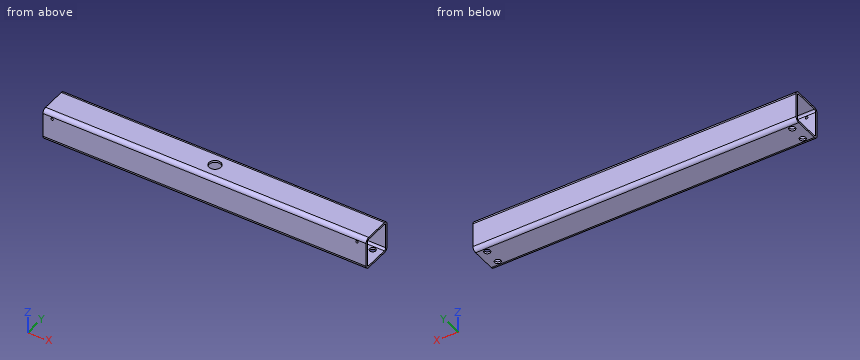
```python
from build123d import *

# Parameters (mm, degrees)
BASE_EXTRUDE_DEPTH = 511.175
SKETCH3_R          = 19.05
CUT_EXTRUDE1_DEPTH = 25.4
SKETCH4_R          = 9.525
CUT_EXTRUDE2_DEPTH = 25.4
SKETCH5_R          = 3.9751
CUT_EXTRUDE3_DEPTH = 25.4


with BuildPart() as part:
    # Sketch1 → Base-Extrude (new, symmetric)
    with BuildSketch(Plane(origin=(0, 0, 0), x_dir=(0, 0, -1), z_dir=(1, 0, 0))):
        with BuildLine():
            Line((-127, 139.7), (-50.8, 139.7))
            ThreePointArc((-50.8, 139.7), (-41.819743879, 135.980256121), (-38.1, 127))
            Line((-38.1, 127), (-38.1, 50.8))
            ThreePointArc((-38.1, 50.8), (-41.819743879, 41.819743879), (-50.8, 38.1))
            Line((-50.8, 38.1), (-127, 38.1))
            ThreePointArc((-127, 38.1), (-135.980256121, 41.819743879), (-139.7, 50.8))
            Line((-139.7, 50.8), (-139.7, 127))
            ThreePointArc((-139.7, 127), (-135.980256121, 135.980256121), (-127, 139.7))
        make_face()
        with BuildLine():
            Line((-127, 133.35), (-50.8, 133.35))
            ThreePointArc((-50.8, 133.35), (-46.309871939, 131.490128061), (-44.45, 127))
            Line((-44.45, 127), (-44.45, 50.8))
            ThreePointArc((-44.45, 50.8), (-46.309871939, 46.309871939), (-50.8, 44.45))
            Line((-50.8, 44.45), (-127, 44.45))
            ThreePointArc((-127, 44.45), (-131.490128061, 46.309871939), (-133.35, 50.8))
            Line((-133.35, 50.8), (-133.35, 127))
            ThreePointArc((-133.35, 127), (-131.490128061, 131.490128061), (-127, 133.35))
        make_face(mode=Mode.SUBTRACT)
    extrude(amount=BASE_EXTRUDE_DEPTH, both=True)

    # Sketch3 → Cut-Extrude1 (cut)
    with BuildSketch(Plane.XY.offset(139.7)):
        with Locations((0, 88.9)):
            Circle(SKETCH3_R)
    extrude(amount=-CUT_EXTRUDE1_DEPTH, mode=Mode.SUBTRACT)

    # Sketch4 → Cut-Extrude2 (cut)
    with BuildSketch(Plane(origin=(0, 0, 38.1), x_dir=(-1, 0, 0), z_dir=(0, 0, -1))):
        with Locations(Location((-482.6, 63.5, 0), (0, 0, 90))):
            Circle(SKETCH4_R)
        with Locations(Location((-482.6, 114.3, 0), (0, 0, 90))):
            Circle(SKETCH4_R)
    cut_extrude2 = extrude(amount=-CUT_EXTRUDE2_DEPTH, mode=Mode.SUBTRACT)

    # Sketch5 → Cut-Extrude3 (cut)
    with BuildSketch(Plane.XZ.offset(-38.1)):
        with Locations(Location((482.6, 120.65, 0), (0, 0, 270))):
            Circle(SKETCH5_R)
    cut_extrude3 = extrude(amount=-CUT_EXTRUDE3_DEPTH, mode=Mode.SUBTRACT)

    # Mirror1: Cut-Extrude2, Cut-Extrude3 across plane
    add(cut_extrude2.mirror(Plane(origin=(0, 0, 0), x_dir=(0, 0, 1), z_dir=(1, 0, 0))), mode=Mode.SUBTRACT)
    add(cut_extrude3.mirror(Plane(origin=(0, 0, 0), x_dir=(0, 0, 1), z_dir=(1, 0, 0))), mode=Mode.SUBTRACT)


solid = part.part
```
Verification items for the finished model (mm, model axes). Give positions to 0.01 mm unless a question says otherwise; leave off trailing zeros. Order: outer loops, then holes, each group sorted by start corner. A loop starts at its lowest first (then second) coordinate and runs counter-clockwise, first axis right, second up. Notation, with made-up numbers: (37.5, 15.5) -> (62.5, 15.5) arc R8 cw to (62.5, 23.5) -> close; hole circle Ø9 at (19.5, -24.75). An arc over 180 degrees is marked (long way). One line per item, written item: value.
(1) Scan lines: line 1 along X through (y, z) = (63.5, 42.5) (3 decimals); line 2 along Y through (x, z) = (-211, 107). Record each from-to range of solid material in increasing order. Write a range as [from, to].
Final values:
line 1: [-511.175, -492.125], [-473.075, 473.075], [492.125, 511.175]
line 2: [38.1, 44.45], [133.35, 139.7]
(2) Gauge pin test, flat end, axial feed: pin 1 (17 mm diameter, centred on x = 482.6, y = 63.5, fed in from -Z). Record the tip position at first contact, or that the pin passes through.
Final values:
pin 1: z = 133.35
(3) Sectioned sample at B-B on y = 88.9. Record the cut outline in (x, z) (3 decimals), then the cut area to 3 significant figures.
Final values:
outline: (-511.175, 38.1) -> (511.175, 38.1) -> (511.175, 44.45) -> (-511.175, 44.45) -> close; (-511.175, 133.35) -> (-19.05, 133.35) -> (-19.05, 139.7) -> (-511.175, 139.7) -> close; (19.05, 133.35) -> (511.175, 133.35) -> (511.175, 139.7) -> (19.05, 139.7) -> close
area: 12,700 mm^2
(4) Sectioned sample at D-D on x = 0. Record the cut outline in (y, z), then the cut area to 3 significant figures.
Final values:
outline: (38.1, 50.8) arc R12.7 ccw to (50.8, 38.1) -> (127, 38.1) arc R12.7 ccw to (139.7, 50.8) -> (139.7, 127) arc R12.7 ccw to (127, 139.7) -> (107.95, 139.7) -> (107.95, 133.35) -> (127, 133.35) arc R6.35 cw to (133.35, 127) -> (133.35, 50.8) arc R6.35 cw to (127, 44.45) -> (50.8, 44.45) arc R6.35 cw to (44.45, 50.8) -> (44.45, 127) arc R6.35 cw to (50.8, 133.35) -> (69.85, 133.35) -> (69.85, 139.7) -> (50.8, 139.7) arc R12.7 ccw to (38.1, 127) -> close
area: 2,070 mm^2
(5) Sectioned sample at A-A on z = 87.5. Record the cut outline in (x, y) (3 decimals).
Final values:
outline: (-511.175, 38.1) -> (511.175, 38.1) -> (511.175, 44.45) -> (-511.175, 44.45) -> close; (-511.175, 133.35) -> (511.175, 133.35) -> (511.175, 139.7) -> (-511.175, 139.7) -> close
(6) Sectioned sample at C-C on x = -273. Record the cut outline in (y, z), then the cut area to 3 significant figures.
Final values:
outline: (38.1, 50.8) arc R12.7 ccw to (50.8, 38.1) -> (127, 38.1) arc R12.7 ccw to (139.7, 50.8) -> (139.7, 127) arc R12.7 ccw to (127, 139.7) -> (50.8, 139.7) arc R12.7 ccw to (38.1, 127) -> close; hole (44.45, 50.8) arc R6.35 ccw to (50.8, 44.45) -> (127, 44.45) arc R6.35 ccw to (133.35, 50.8) -> (133.35, 127) arc R6.35 ccw to (127, 133.35) -> (50.8, 133.35) arc R6.35 ccw to (44.45, 127) -> close
area: 2,320 mm^2
